Model file for the job. Use its own axes, mm. A direction names the side the tool comes from. Give positions to 0.01 mm unless a question says otherwise; leave off trailing zeros. Loops run counter-clockwise (first coordinate to the right, second up) from the corner with the lowest first, then second, coordinate; pieces in that order, holes last. Notation, with made-up numbers: (-17.75, 48.25) -> (9.25, 48.25) arc R19 ccw to (9.25, 55.25) -> close; hole circle Ø3 at (80, 14). An arc over 180 degrees is marked (long way). Use CSV: the item, a comma, the result in double quotes. Start each with the question number.
(1) Cut at B-B on z = 7.5. Write the cut outline in (x, y).
(2) Pull direction X, two halves, no side cores. Call faces 4 (the flat face through (-6, 40, 3)), 5 (the flat face through (-6.5, 37, 3)), 6 (the flat face through (6.5, 38, 3)), 7 (the flat face through (0, 37, 3)): pulls with the +X half, pulls with the -X half, needs draft (parallel to the pull), parting line crosses it, or undercut.
(3) Cut at A-A on y = 39.4. Write the cut outline in (x, z), then the cut area to 3 significant figures.
(4) Cut at D-D on z = 4.5. Write the cut outline in (x, y).
(5) Drill centre lines: probe 1 along X at (y, z) = (38.3, 2.25); probe 2 along Y at (x, z) = (-2, 0.5); probe 3 along Y at (x, z) = (4.25, 7). Where is each one in solid material? Low to high.
(6) Cut at C-C on x = 0.5. Write the cut outline in (y, z), then the cut area to 3 significant figures.
(7) Flat gauge pins, fed straight in: pin 1 (1 mm diameter, centred on x = 1.5, z = 7.5, fed in from -Y); pin 2 (2 mm diameter, centred on x = 1.5, z = 5.5, fed in from +Y). Where does each tip first touch, or does it go through?
(8) 3-axis set-ups, long thin cutter, end or side, ignore diameter. For faces 1 (the flat face through (-5.5, 39, 3)), 2 (the flat face through (0, 35, 2)), 3 (the flat face through (0.1, 35.5, 6)): which of +Z, -Z, +X, -X, +Y, -Y reach the whole face in a straight line?
from build123d import *

# Parameters (mm, degrees)
SKETCH050_W      = 2
SKETCH050_H      = 3
EXTRUDE047_DEPTH = 7
EXTRUDE046_DEPTH = 9


with BuildPart() as extrude047:
    # Sketch050 → Extrude047 (new body, symmetric)
    with BuildSketch(Plane.YZ):
        with Locations((35.1, 7.5)):
            Rectangle(SKETCH050_W, SKETCH050_H)
    extrude(amount=EXTRUDE047_DEPTH, both=True)


with BuildPart() as cut040:
    # Sketch049 → Extrude046 (new body)
    with BuildSketch(Plane.XY.offset(-1)):
        Polygon((-5.5, 40), (-5.5, 37), (5.5, 37), (5.5, 40), (6.5, 40), (6.5, 35), (-6.5, 35), (-6.5, 40), align=None)
    extrude(amount=EXTRUDE046_DEPTH)

    # Cut040: cut Extrude047
    add(extrude047.part, mode=Mode.SUBTRACT)


solid = cut040.part
Check result:
1,outline,"(-6.5, 36.1) -> (6.5, 36.1) -> (6.5, 40) -> (5.5, 40) -> (5.5, 37) -> (-5.5, 37) -> (-5.5, 40) -> (-6.5, 40) -> close"
2,face 4,"needs draft"
2,face 5,"pulls with the -X half"
2,face 6,"pulls with the +X half"
2,face 7,"undercut"
3,outline,"(-6.5, -1) -> (-5.5, -1) -> (-5.5, 8) -> (-6.5, 8) -> close; (5.5, -1) -> (6.5, -1) -> (6.5, 8) -> (5.5, 8) -> close"
3,area,"18.0 mm²"
4,outline,"(-6.5, 35) -> (6.5, 35) -> (6.5, 40) -> (5.5, 40) -> (5.5, 37) -> (-5.5, 37) -> (-5.5, 40) -> (-6.5, 40) -> close"
5,probe 1,"-6.5 to -5.5, 5.5 to 6.5"
5,probe 2,"35 to 37"
5,probe 3,"36.1 to 37"
6,outline,"(35, -1) -> (37, -1) -> (37, 8) -> (36.1, 8) -> (36.1, 6) -> (35, 6) -> close"
6,area,"15.8 mm²"
7,pin 1,"y = 36.1"
7,pin 2,"y = 37"
8,face 1,"+Z, -Z, +Y"
8,face 2,"+Z, -Z, +X, -X, -Y"
8,face 3,"+Z, +X, -X, -Y"
